Design review of the part built by this model. Coordinates are the model's own, in mm. A direction names the side the tool comes from. Coordinates: 2 decimals unless noted, no trailing zeros. Write each loop counter-clockwise with the first axis right and the second up, starting at its lowest first coordinate (ties: lowest second). Pieces come first, ordered by that corner, then holes. Notation, with made-up numbers: M -24.5,56.25 L -6.5,56.25 A33 ccw -6.5,84.25 Z; hole C -21,1 d9. An arc over 180 degrees is marked long. Write each question's results on one line, items separated by ' | '. Start each with the question number.
Autodesk Inventor part; units mm, degrees
ref_plane "YZ Plane" through (0, 0, 0) normal (1, 0, 0) x (0, 1, 0)
ref_plane "XZ Plane" through (0, 0, 0) normal (0, 1, 0) x (-1, 0, 0)
ref_plane "XY Plane" through (0, 0, 0) normal (0, 0, 1) x (1, 0, 0)
sketch "Sketch1" plane through (0, 0, 0) normal (0, 0, 1) x (1, 0, 0)
  line L0 (-4.8549, 2.8898) -> (4.6751, 2.8898)
  line L1 (4.6751, 2.8898) -> (4.6751, -6.6402)
  line L2 (4.6751, -6.6402) -> (-4.8549, -6.6402)
  line L3 (-4.8549, -6.6402) -> (-4.8549, 2.8898)
  point P0 (0, 0)
  dimension "d0" = 9.53
  dimension "d1" = 9.53
extrude "Extrusion1" add sketch "Sketch1" along normal blind 1.65
sketch "Sketch2" plane through (4.6751, -6.6402, 0) normal (1, 0, 0) x (0, 0, -1)
  line L0 (-1.65, 0) -> (-1.65, 9.53)
  line L1 (-1.65, 3.59) -> (-6.4, 3.59)
  line L2 (-6.4, 3.59) -> (-6.4, 4.61)
  line L3 (-6.4, 4.61) -> (-1.65, 4.61)
  line L4 (-1.65, 4.61) -> (-1.65, 3.59)
  line L5 (-1.65, 0) -> (-6.4, 0)
  line L6 (-6.4, 0) -> (-6.4, 1.91)
  line L7 (-6.4, 1.91) -> (-1.65, 1.91)
  line L8 (-1.65, 1.91) -> (-1.65, 0)
  point P0 (0, 6.6402)
  dimension "d4" = 1.68
  dimension "d5" = 1.91
  dimension "d6" = 1.02
  dimension "d7" = 4.75
  dimension "d8" = 4.75
extrude "Extrusion2" add sketch "Sketch2" against normal blind 9.53
sketch "Sketch3" plane through (0, 0, 0) normal (0, 0, -1) x (-1, 0, 0)
  circle A0 centre (0, -1.8752) radius 3.05
  point P0 (0, 0)
  dimension "d11" = 6.1
extrude "Extrusion3" add sketch "Sketch3" along normal blind 7.88
properties part number "SMA_Edge"
Item 1: We need section A-A on z = 4.5. State the section outline as (x, y) points, then the cut area to 3 significant figures.
Item 2: We need section B-B on x = 0. State the section outline as (y, z) points.
Item 3: Draft analysis for pull direction Y (two halves, no side actions). For faces 5 (the flat face through (0, -4, 1.65)), 6 (the flat face through (0, -2, -7.88)), 7 (the flat face through (0, -6.64, 3)), state which applies: released by +Y, released by -Y, zero draft, split by the parting line, or undercut.
Item 4: Wall thickness on L1, parallel to Y at x = 4.25, z = 4.5; L2, parallel to Z at x = 1, y = 0.75; L3, parallel to Z at x = -3, y = -4: over which ranges is each line inside the solid? List them lowest first.
Item 5: Insertion check: pin 1 Ø3 at (y, z) = (-4.5, -4.5) entering from -X (3 decimals); pin 2 Ø1 at (y, z) = (-0.5, -3) entering from +X; pin 3 Ø1.5 at (x, y) = (1, -0.5) entering from +Z. Each pin has a flat end and moves straight along its axis. Give the tip position at first contact, or say it passes through.
Item 6: For faces 1 (the flat face through (4.675, -2.9, 2.4)), 2 (the flat face through (0, -2.03, 4)), 3 (the flat face through (-3.3, -1.8, 0)), 4 (the flat face through (0, -3.05, 4)), list the 3-axis set-ups (+Z, -Z, +X, -X, +Y, -Y) from which the entire face can be reached by the end or side of a thin tool; tool diameter is ignored.
Item 7: We need section C-C on y = -4.5. State the section outline as (x, z) points, then the cut area to 3 significant figures.
Item 8: We need section D-D on x = -2.5. State the section outline as (y, z) points, then the cut area to 3 significant figures.
Answer:
1) outline: M -4.85,-6.64 L 4.68,-6.64 L 4.68,-4.73 L -4.85,-4.73 Z; M -4.85,-3.05 L 4.68,-3.05 L 4.68,-2.03 L -4.85,-2.03 Z | area: 27.9 mm^2
2) outline: M -6.64,0 L -4.93,0 L -4.93,-7.88 L 1.17,-7.88 L 1.17,0 L 2.89,0 L 2.89,1.65 L -2.03,1.65 L -2.03,6.4 L -3.05,6.4 L -3.05,1.65 L -4.73,1.65 L -4.73,6.4 L -6.64,6.4 Z
3) face 5: undercut | face 6: zero draft | face 7: released by -Y
4) L1: y = -6.64 to -4.73, -3.05 to -2.03 | L2: z = -7.88 to 1.65 | L3: z = 0 to 1.65
5) pin 1: stops at x = -2.835 | pin 2: stops at x = 2.92 | pin 3: stops at z = 1.65
6) face 1: +Z, -Z, +X, +Y, -Y | face 2: +Z, +X, -X, +Y | face 3: -Z | face 4: +Z, +X, -X
7) outline: M -4.85,0 L -1.55,0 L -1.55,-7.88 L 1.55,-7.88 L 1.55,0 L 4.68,0 L 4.68,1.65 L -4.85,1.65 Z | area: 40.2 mm^2
8) outline: M -6.64,0 L -3.62,0 L -3.62,-7.88 L -0.13,-7.88 L -0.13,0 L 2.89,0 L 2.89,1.65 L -2.03,1.65 L -2.03,6.4 L -3.05,6.4 L -3.05,1.65 L -4.73,1.65 L -4.73,6.4 L -6.64,6.4 Z | area: 57.2 mm^2
